```python
from build123d import *

# Parameters (mm, degrees)
BOSS_EXTRUDE1_DEPTH  = 3
M4_CLEARANCE_HOLE1_D = 4.5


with BuildPart() as part:
    # Sketch1 → Boss-Extrude1 (new body)
    with BuildSketch(Plane.XY):
        Polygon((31.645266951, 0), (474.645266951, 0), (474.645266951, 26), (500.645266951, 26), (500.645266951, 149), (449.645266951, 149), (449.645266951, 175), (56.645266951, 175), (56.645266951, 149), (5.645266951, 149), (5.645266951, 26), (31.645266951, 26), align=None)
    extrude(amount=BOSS_EXTRUDE1_DEPTH)

    # M4 Clearance Hole1 (through all)
    with Locations(Plane.XY.offset(3)):
        with Locations((253.145266951, 12.5), (253.145266951, 162.5), (437.145266951, 12.5), (437.145266951, 162.5), (69.145266951, 162.5), (69.145266951, 12.5)):
            Hole(M4_CLEARANCE_HOLE1_D / 2)


solid = part.part
```
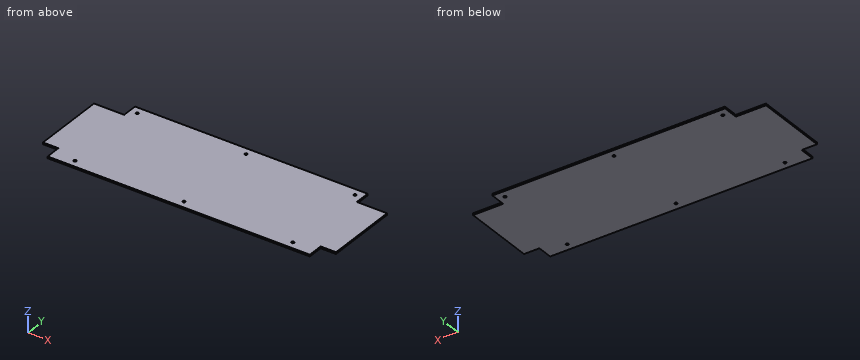
Part model, mm, in its own coordinate system. Round coordinates to 2 decimals unless told otherwise and drop trailing zeros. Loops run counter-clockwise (first coordinate to the right, second up) from the corner with the lowest first, then second, coordinate; pieces in that order, holes last. Notation, with made-up numbers: (40.25, 74.25) -> (92.25, 74.25) arc R18 ccw to (92.25, 93.25) -> close; hole circle Ø5 at (-19, -19.5). An arc over 180 degrees is marked (long way). Use a Markdown table: item, result.
1) Probe line 1 (X direction, y = 162.5, z = 1.3); line 2 (X direction, y = 16.5, z = 1.5); line 3 (X direction, y = 149.5, z = 2.45). List the from-to ranges inside material, lowest first. Write a range as [from, to].
The answers:
| item | result |
|---|---|
| line 1 | x = [56.65, 66.9], [71.4, 250.9], [255.4, 434.9], [439.4, 449.65] |
| line 2 | x = [31.65, 474.65] |
| line 3 | x = [56.65, 449.65] |
2) Cut at A-A, the plane z = 1.1. List the corners of the cut face in (x, y), and give its area (3 significant figures).
The answers:
| item | result |
|---|---|
| outline | (5.65, 26) -> (31.65, 26) -> (31.65, 0) -> (474.65, 0) -> (474.65, 26) -> (500.65, 26) -> (500.65, 149) -> (449.65, 149) -> (449.65, 175) -> (56.65, 175) -> (56.65, 149) -> (5.65, 149) -> close; hole circle Ø4.5 at (69.15, 12.5); hole circle Ø4.5 at (69.15, 162.5); hole circle Ø4.5 at (253.15, 12.5); hole circle Ø4.5 at (253.15, 162.5); hole circle Ø4.5 at (437.15, 12.5); hole circle Ø4.5 at (437.15, 162.5) |
| area | 82,500 mm2 |
3) Drop flat-ended pins along their axis: pin 1 Ø1.5 at (y, z) = (13, 1) entering from -X; pin 2 Ø1.5 at (y, z) = (164.5, 1.5) entering from +X; pin 3 Ø1.5 at (y, z) = (17, 1) entering from +X; pin 4 Ø3.5 at (x, y) = (437.15, 162.5) entering from -Z. Give the stop position or say it passes through.
The answers:
| item | result |
|---|---|
| pin 1 | stops at x = 31.65 |
| pin 2 | stops at x = 449.65 |
| pin 3 | stops at x = 474.65 |
| pin 4 | passes through |
4) Cut at B-B, the plane x = 461. List the corners of the cut face in (y, z), and give its area (3 significant figures).
The answers:
| item | result |
|---|---|
| outline | (0, 0) -> (149, 0) -> (149, 3) -> (0, 3) -> close |
| area | 447 mm2 |
